Geometry check sheet. Reference: the model listing, model coordinates, mm. Coordinates: 2 decimals unless noted, no trailing zeros. Write each loop counter-clockwise with the first axis right and the second up, starting at its lowest first coordinate (ties: lowest second). Pieces come first, ordered by that corner, then holes. Notation, with made-up numbers: (20, 20) -> (68, 20) arc R14 cw to (68, 26) -> close; hole circle Ø5 at (-11.5, 41.25). An arc over 180 degrees is marked (long way). Answer in a Markdown table with one row per item. Add a question column.
Q1. Thickness scan on line 1 (Z direction, x = 0, y = -349.5); line 2 (Y direction, x = -0.75, z = -2); line 3 (X direction, y = -112, z = -1). Record the ranges inside material, lowest first.
Q2. Section check A-A, the plane z = 0. Record the boundary of the cut face in (x, y).
Q3. Section check B-B, the plane x = 0. Record the boundary of the cut face in (y, z), and give its area (3 significant figures).
Q4. Section check C-C, the plane y = -274. Record the boundary of the cut face in (x, z).
Q5. Gauge pin test, flat ends, axial feed: P1, Ø2.5, axis at x = -1.5, z = -2, coming from the -Y side; P2, Ø1, axis at x = 7, y = -247.5, coming from the -Z side; P3, Ø1, axis at x = 2, y = -264, coming from the +Z side. Record the tip position at first contact, or that the pin passes through.
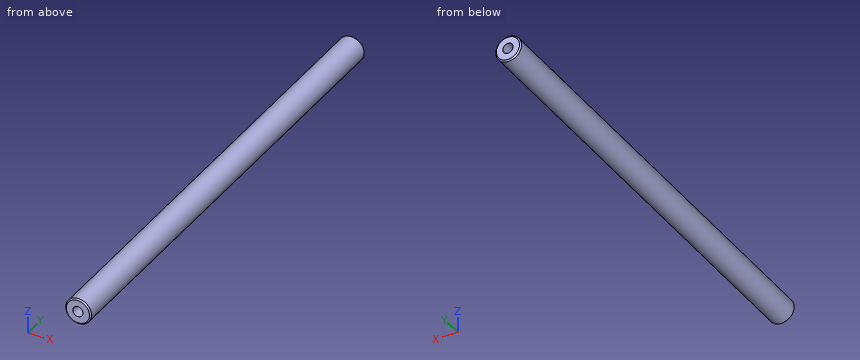
```python
from build123d import *

# Parameters (mm, degrees)
F0_R     = 10
F1_DEPTH = 366
F2_SIZE  = 1
F3_R     = 4
F4_DEPTH = 25
F5_R     = 4
F6_DEPTH = 25


with BuildPart() as f1:
    # F0 (on Front) → F1 (new body)
    with BuildSketch(Plane.XZ):
        Circle(F0_R)
    extrude(amount=F1_DEPTH)

    # F2
    f2_edges = [f1.edges().sort_by_distance(p)[0] for p in [
        (-10, -366, 0),
        (-10, 0, 0),
    ]]
    chamfer(f2_edges, length=F2_SIZE)

    # F3 (on face) → F4 (cut)
    with BuildSketch(Plane.XZ.offset(366)):
        Circle(F3_R)
    extrude(amount=-F4_DEPTH, mode=Mode.SUBTRACT)

    # F5 (on face) → F6 (cut)
    with BuildSketch(Plane(origin=(0, 0, 0), x_dir=(-1, 0, 0), z_dir=(0, 1, 0))):
        Circle(F5_R)
    extrude(amount=-F6_DEPTH, mode=Mode.SUBTRACT)


solid = f1.part
```
Calculated:
| question | item | result |
|---|---|---|
| 1 | line 1 | z = -10 to -4, 4 to 10 |
| 1 | line 2 | y = -341 to -25 |
| 1 | line 3 | x = -9.95 to 9.95 |
| 2 | outline | (-10, -365) -> (-9, -366) -> (-4, -366) -> (-4, -341) -> (4, -341) -> (4, -366) -> (9, -366) -> (10, -365) -> (10, -1) -> (9, 0) -> (4, 0) -> (4, -25) -> (-4, -25) -> (-4, 0) -> (-9, 0) -> (-10, -1) -> close |
| 3 | outline | (-366, -9) -> (-365, -10) -> (-1, -10) -> (0, -9) -> (0, -4) -> (-25, -4) -> (-25, 4) -> (0, 4) -> (0, 9) -> (-1, 10) -> (-365, 10) -> (-366, 9) -> (-366, 4) -> (-341, 4) -> (-341, -4) -> (-366, -4) -> close |
| 3 | area | 6,920 mm² |
| 4 | outline | circle Ø20 at (0, 0) |
| 5 | P1 | stops at y = -341 |
| 5 | P2 | stops at z = -7.6 |
| 5 | P3 | stops at z = 9.89 |
